```python
from build123d import *

# Parameters (mm, degrees)
SKETCH2_R               = 1.4
SKETCH2_R_2             = 1.535241885
SKETCH2_W               = 23.4
SKETCH2_H               = 13
BOSS_EXTRUDE2_DEPTH     = 4
CUT_EXTRUDE3_DEPTH      = 48.403797316
CUT_EXTRUDE3_DEPTH_BACK = 48.403797316
SKETCH3_R               = 2.5
FILLET1_R               = 1


with BuildPart() as part:
    # Sketch2 → Boss-Extrude2 (new body)
    with BuildSketch(Plane(origin=(0, 0, 0), x_dir=(1, 0, 0), z_dir=(0, 1, 0))):
        with BuildLine():
            Line((29, 4.4), (7.95, 4.4))
            Line((7.95, 4.4), (7.95, 8.5))
            Line((7.95, 8.5), (4.4, 8.5))
            Line((4.4, 8.5), (4.4, 29))
            ThreePointArc((4.4, 29), (0, 33.4), (-4.4, 29))
            Line((-4.4, 29), (-4.4, 8.5))
            Line((-4.4, 8.5), (-22.65, 8.5))
            Line((-22.65, 8.5), (-22.65, 4.4))
            Line((-22.65, 4.4), (-29, 4.4))
            ThreePointArc((-29, 4.4), (-33.4, 0), (-29, -4.4))
            Line((-29, -4.4), (-22.65, -4.4))
            Line((-22.65, -4.4), (-22.65, -8.5))
            Line((-22.65, -8.5), (-4.4, -8.5))
            Line((-4.4, -8.5), (-4.4, -29))
            ThreePointArc((-4.4, -29), (0, -33.4), (4.4, -29))
            Line((4.4, -29), (4.4, -8.5))
            Line((4.4, -8.5), (7.95, -8.5))
            Line((7.95, -8.5), (7.95, -4.4))
            Line((7.95, -4.4), (29, -4.4))
            ThreePointArc((29, -4.4), (33.4, 0), (29, 4.4))
        make_face()
        with Locations(Location((0, 29, 0), (0, 0, 270))):
            Circle(SKETCH2_R, mode=Mode.SUBTRACT)
        with Locations(Location((29, 0, 0), (0, 0, 270))):
            Circle(SKETCH2_R, mode=Mode.SUBTRACT)
        with Locations(Location((0, -29, 0), (0, 0, 90))):
            Circle(SKETCH2_R, mode=Mode.SUBTRACT)
        with Locations(Location((-29, 0, 0), (0, 0, 90))):
            Circle(SKETCH2_R, mode=Mode.SUBTRACT)
        with Locations(Location((6.5, 0, 0), (0, 0, 270))):
            Circle(SKETCH2_R_2, mode=Mode.SUBTRACT)
        with Locations(Location((-21.2, 0, 0), (0, 0, 270))):
            Circle(SKETCH2_R_2, mode=Mode.SUBTRACT)
        with Locations((-7.35, 0)):
            Rectangle(SKETCH2_W, SKETCH2_H, mode=Mode.SUBTRACT)
    extrude(amount=BOSS_EXTRUDE2_DEPTH)

    # Sketch3 → Cut-Extrude3 (cut, two sides: drawn at the far end of the back side and taken through both)
    with BuildSketch(Plane(origin=(0, 0, 0), x_dir=(1, 0, 0), z_dir=(0, 1, 0)).offset(-CUT_EXTRUDE3_DEPTH_BACK)):
        with Locations(Location((0, 21.25, 0), (0, 0, 270))):
            Circle(SKETCH3_R)
        with Locations(Location((0, 14.25, 0), (0, 0, 270))):
            Circle(SKETCH3_R)
        with Locations(Location((14.25, 0, 0), (0, 0, 270))):
            Circle(SKETCH3_R)
        with Locations(Location((21.25, 0, 0), (0, 0, 270))):
            Circle(SKETCH3_R)
        with Locations(Location((0, -14.25, 0), (0, 0, 270))):
            Circle(SKETCH3_R)
        with Locations(Location((0, -21.25, 0), (0, 0, 270))):
            Circle(SKETCH3_R)
    extrude(amount=CUT_EXTRUDE3_DEPTH + CUT_EXTRUDE3_DEPTH_BACK, mode=Mode.SUBTRACT)

    # Fillet1
    fillet1_edges = [part.edges().sort_by_distance(p)[0] for p in [
        (7.95, 2, 4.4),
        (7.95, 2, 8.5),
        (4.4, 2, 8.5),
        (-4.4, 2, 8.5),
        (-22.65, 2, 8.5),
        (-22.65, 2, 4.4),
        (-22.65, 2, -4.4),
        (-22.65, 2, -8.5),
        (-4.4, 2, -8.5),
        (4.4, 2, -8.5),
        (7.95, 2, -8.5),
        (7.95, 2, -4.4),
    ]]
    fillet(fillet1_edges, radius=FILLET1_R)


solid = part.part
```
Input: part model. Units: mm. Frame: model coordinates. A direction names the side the tool comes from. Round coordinates to 2 decimals unless told otherwise and drop trailing zeros. Loops run counter-clockwise (first coordinate to the right, second up) from the corner with the lowest first, then second, coordinate; pieces in that order, holes last. Notation, with made-up numbers: (81.5, 49.5) - (86.5, 49.5) arc R29 ccw to (86.5, 74.5) - close; hole circle Ø9 at (-13, -34). An arc over 180 degrees is marked (long way). One line per item, written item: value. Start each with the question number.
(1) Contact query for flat-ended pins moving along their axis: P1, Ø1.2, axis at y = 2, z = -19.5, coming from the +X side; P2, Ø1.7, axis at x = 6, y = 2, coming from the -Z side; P3, Ø1.2, axis at x = 6, y = 2, coming from the +Z side. Output: stop coordinate, or through.
(2) Ray query, line 1 (X direction, y = 1.1, z = 21.25); line 2 (X direction, y = 2.4, z = -29). Return the intervals inside material, ascending. Write a range as [from, to].
(3) Draft query along X for faces 6 (the cylindrical face through (0.11, 1.972, -16.748)), 7 (the flat face through (19, 2, 4.4)), 8 (the flat face through (-4.4, 2, -19)), 9 (the cylindrical face through (23.73, 1.97, -0.33)). Return one class per face: +X half, -X half, draft (parallel to the pull), parting line (faces both ways), or undercut.
(4) Section C-C, the plane x = 21.25. Return loops of the section in (y, z).
(5) Access query for faces 1 (the flat face through (-13, 2, -8.5)), 2 (the flat face through (-19.05, 2, 0)), 3 (the flat face through (6, 2, 8.5)), 4 (the flat face through (-4.4, 2, 19)), 5 (the flat face through (6, 2, -8.5)). Directions: +Z, -Z, +X, -X, +Y, -Y. A direction counts if a zero-diameter tool reaches every point of the face in a straight line with its end or side. Return the directions, or none.
(6) Section B-B, the plane z = 14.25. Return loops of the section in (x, y).
(7) Section A-A, the plane x = 0. Count the separate pieces of the cut face and the enclosed holes in it, plus the area to 3 significant figures.
Results below:
1. P1: x = 4.4
1. P2: z = -8.53
1. P3: z = 8.5
2. line 1: [-4.4, -2.5], [2.5, 4.4]
2. line 2: [-4.4, -1.4], [1.4, 4.4]
3. face 6: undercut
3. face 7: draft
3. face 8: -X half
3. face 9: undercut
4. outline: (0, -4.4) - (4, -4.4) - (4, -2.5) - (0, -2.5) - close; (0, 2.5) - (4, 2.5) - (4, 4.4) - (0, 4.4) - close
5. face 1: -Z, -X, +Y, -Y
5. face 2: +Y, -Y
5. face 3: +Z, +X, +Y, -Y
5. face 4: +Z, -X, +Y, -Y
5. face 5: -Z, +X, +Y, -Y
6. outline: (-4.4, 0) - (-2.5, 0) - (-2.5, 4) - (-4.4, 4) - close; (2.5, 0) - (4.4, 0) - (4.4, 4) - (2.5, 4) - close
7. separate pieces: 8
7. enclosed holes: 0
7. area: 113 mm^2
